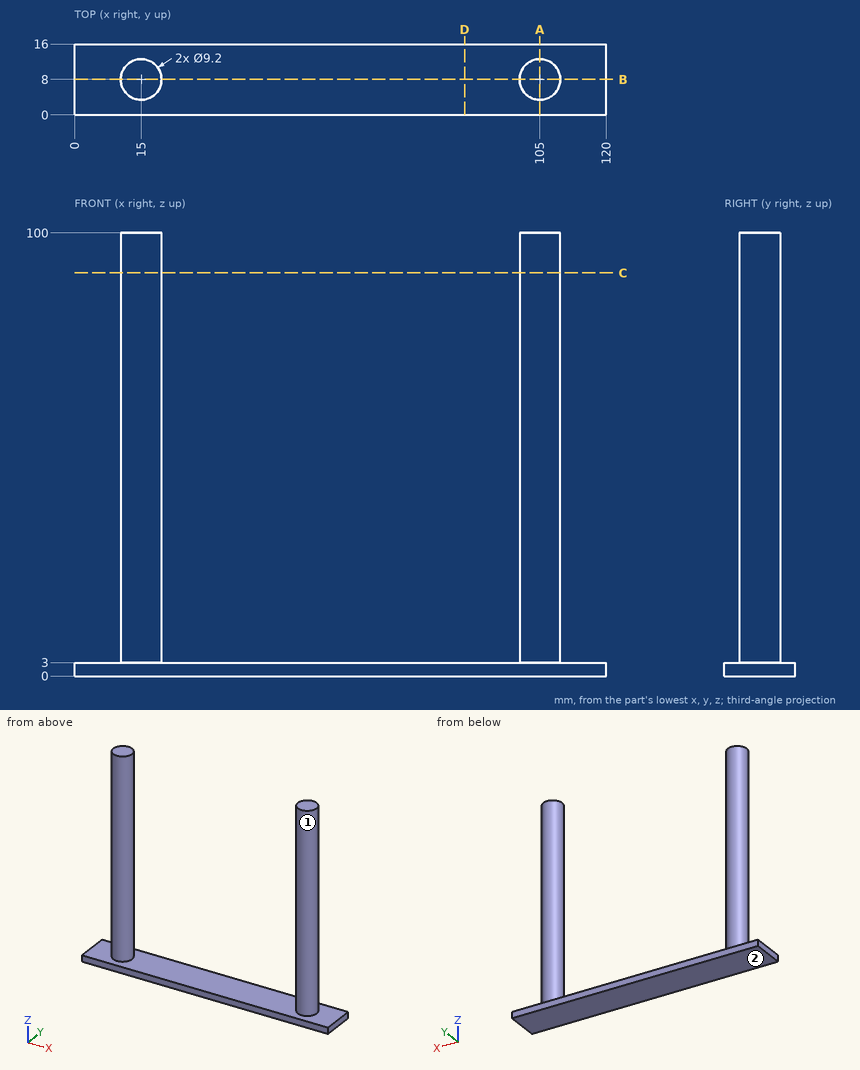
Source: three-view drawing plus pictorial views. Frame: mm from the lowest corner of the part. A direction names the side the tool comes from. Round coordinates to 2 decimals unless told otherwise and drop trailing zeros. Loops run counter-clockwise (first coordinate to the right, second up) from the corner with the lowest first, then second, coordinate; pieces in that order, holes last. Notation, with made-up numbers: (44, -32.5) - (54, -32.5) arc R26 ccw to (54, -5.5) - close; hole circle Ø6 at (-22, -2.5). An arc over 180 degrees is marked (long way). Write each question's results on one line, items separated by ' | '. Start each with the question number.
1) Access query for the marked faces 1 and 2. Directions: +Z, -Z, +X, -X, +Y, -Y. A direction counts if a zero-diameter tool reaches every point of the face in a straight line with its end or side. Return the directions, or none.
2) Cut plane C-C on z = 91. Return loops of the section in (x, y).
3) Cut plane B-B on y = 8. Return loops of the section in (x, z), then the cut area to 3 significant figures.
4) First-contact query: P1, Ø1.5, axis at x = 89.5, y = 7, coming from the +Z side; P2, Ø2, axis at y = 9, z = 43.5, coming from the +X side; P3, Ø12, axis at x = 16, z = 79.5, coming from the +Y side. Flat tips, straight axial feed; report the tip coordinate or a pass-through.
5) Cut plane D-D on x = 88. Return loops of the section in (y, z).
6) Cut plane A-A on x = 105. Return loops of the section in (y, z).
7) Line query: probe 1 along Z at (x, y) = (60, 2.25); probe 2 along X at (y, z) = (8, 85); probe 3 along X at (y, z) = (6.25, 78.5). Output: solid intervals per line, ascending. Write a range as [from, to].
Verdict:
1) face 1: +Z | face 2: -Z, +X, -X, +Y, -Y
2) outline: circle Ø9.2 at (15, 8); circle Ø9.2 at (105, 8)
3) outline: (0, 0) - (120, 0) - (120, 3) - (109.6, 3) - (109.6, 100) - (100.4, 100) - (100.4, 3) - (19.6, 3) - (19.6, 100) - (10.4, 100) - (10.4, 3) - (0, 3) - close | area: 2,140 mm2
4) P1: stops at z = 3 | P2: stops at x = 109.6 | P3: stops at y = 12.6
5) outline: (0, 0) - (16, 0) - (16, 3) - (0, 3) - close
6) outline: (0, 0) - (16, 0) - (16, 3) - (12.6, 3) - (12.6, 100) - (3.4, 100) - (3.4, 3) - (0, 3) - close
7) probe 1: z = [0, 3] | probe 2: x = [10.4, 19.6], [100.4, 109.6] | probe 3: x = [10.75, 19.25], [100.75, 109.25]
